Design review of the part built by this model. Coordinates are the model's own, in mm. Coordinates: 2 decimals unless noted, no trailing zeros. Write each loop counter-clockwise with the first axis right and the second up, starting at its lowest first coordinate (ties: lowest second). Pieces come first, ordered by that corner, then holes.
Q1. Insertion check: pin 1 (8 mm diameter, centred on x = 33.75, y = 20.18, fed in from +Z). The pin has a flat end and moves straight along its axis. Give the tip position at first contact, or say it passes through.
Q2. Take a section at B-B (x = 33.75). Give the boundary of the cut face in (y, z), and give its area (3 significant figures).
Q3. For probe 1 along Y at (x, z) = (33.75, 2.75); probe 2 along X at (y, z) = (-20.18, 4); probe 3 along Y at (x, z) = (-35.5, 6.25), list the stretches that pass through material, from the lowest coordinate up.
Q4. Take a section at A-A (y = -20.18). Give the boundary of the cut face in (x, z), and give its area (3 significant figures).
Q5. Take a section at C-C (z = 1.5). Give the boundary of the cut face in (x, y), and give its area (3 significant figures).
```python
from build123d import *

# Parameters (mm, degrees)
SKETCH1_W           = 97.5
SKETCH1_H           = 57.36
BOSS_EXTRUDE1_DEPTH = 6.35
SKETCH2_R           = 3
CUT_EXTRUDE1_DEPTH  = 57.915967882


with BuildPart() as part:
    # Sketch1 → Boss-Extrude1 (new body)
    with BuildSketch(Plane.XY):
        Rectangle(SKETCH1_W, SKETCH1_H)
    extrude(amount=BOSS_EXTRUDE1_DEPTH)

    # Sketch2 → Cut-Extrude1 (cut, through all)
    with BuildSketch(Plane.XY.offset(6.35)):
        with Locations((-33.75, 20.18)):
            Circle(SKETCH2_R)
        with Locations((0, 20.18)):
            Circle(SKETCH2_R)
        with Locations((33.75, 20.18)):
            Circle(SKETCH2_R)
        with Locations(Location((33.75, -20.18, 0), (0, 0, 180))):
            Circle(SKETCH2_R)
        with Locations(Location((0, -20.18, 0), (0, 0, 180))):
            Circle(SKETCH2_R)
        with Locations(Location((-33.75, -20.18, 0), (0, 0, 180))):
            Circle(SKETCH2_R)
    extrude(amount=-CUT_EXTRUDE1_DEPTH, mode=Mode.SUBTRACT)


solid = part.part
```
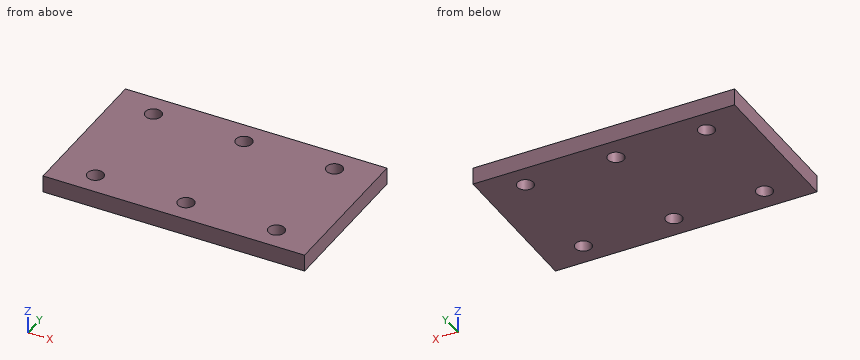
Response:
1. pin 1: stops at z = 6.35
2. outline: (-28.68, 0) - (-23.18, 0) - (-23.18, 6.35) - (-28.68, 6.35) - close; (-17.18, 0) - (17.18, 0) - (17.18, 6.35) - (-17.18, 6.35) - close; (23.18, 0) - (28.68, 0) - (28.68, 6.35) - (23.18, 6.35) - close
2. area: 288 mm2
3. probe 1: y = -28.68 to -23.18, -17.18 to 17.18, 23.18 to 28.68
3. probe 2: x = -48.75 to -36.75, -30.75 to -3, 3 to 30.75, 36.75 to 48.75
3. probe 3: y = -28.68 to -22.62, -17.74 to 17.74, 22.62 to 28.68
4. outline: (-48.75, 0) - (-36.75, 0) - (-36.75, 6.35) - (-48.75, 6.35) - close; (-30.75, 0) - (-3, 0) - (-3, 6.35) - (-30.75, 6.35) - close; (3, 0) - (30.75, 0) - (30.75, 6.35) - (3, 6.35) - close; (36.75, 0) - (48.75, 0) - (48.75, 6.35) - (36.75, 6.35) - close
4. area: 505 mm2
5. outline: (-48.75, -28.68) - (48.75, -28.68) - (48.75, 28.68) - (-48.75, 28.68) - close; hole circle Ø6 at (-33.75, -20.18); hole circle Ø6 at (-33.75, 20.18); hole circle Ø6 at (0, -20.18); hole circle Ø6 at (0, 20.18); hole circle Ø6 at (33.75, -20.18); hole circle Ø6 at (33.75, 20.18)
5. area: 5,420 mm2
